Could you check a few things on this model? Use its own coordinates, in mm. A direction names the side the tool comes from. Coordinates: 2 decimals unless noted, no trailing zeros. Loops run counter-clockwise (first coordinate to the right, second up) from the corner with the lowest first, then second, coordinate; pieces in that order, holes last. Notation, with made-up numbers: (-39, 16.5) -> (-28, 16.5) arc R10 cw to (-28, 28.5) -> close; hole circle Ø2 at (-26, 22.5). An arc over 180 degrees is marked (long way). One line per question, with ' | ' between items.
```python
from build123d import *

# Parameters (mm, degrees)
BOSS_EXTRU_1_DEPTH      = 8
CONG_1_R                = 4
ESQUISSE2_R             = 1.25
ENL_V_MAT_EXTRU_1_DEPTH = 8


with BuildPart() as part:
    # Esquisse1 → Boss.-Extru.1 (new body)
    with BuildSketch(Plane.XY):
        with BuildLine():
            Line((9.8, 25), (4.3, 25))
            Line((4.3, 25), (0, 5))
            Line((0, 5), (0, 0))
            Line((0, 0), (50, 0))
            Line((50, 0), (50, 5))
            Line((50, 5), (45.7, 25))
            Line((45.7, 25), (40.2, 25))
            ThreePointArc((40.2, 25), (25, 9.8), (9.8, 25))
        make_face()
    extrude(amount=BOSS_EXTRU_1_DEPTH)

    # Congé1
    cong_1_edges = [part.edges().sort_by_distance(p)[0] for p in [
        (40.2, 25, 4),
        (9.8, 25, 4),
    ]]
    fillet(cong_1_edges, radius=CONG_1_R)

    # Esquisse2 → Enlèv. mat.-Extru.1 (cut)
    with BuildSketch(Plane.XZ):
        with Locations(Location((5, 4, 0), (0, 0, 270))):
            Circle(ESQUISSE2_R)
        with Locations(Location((45, 4, 0), (0, 0, 90))):
            Circle(ESQUISSE2_R)
    extrude(amount=-ENL_V_MAT_EXTRU_1_DEPTH, mode=Mode.SUBTRACT)


solid = part.part
```
Q1. Imagine slicing it at C-C on x = 45. Write out the boundary of the cut face in (y, z).
Values follow:
outline: (0, 0) -> (25, 0) -> (25, 8) -> (0, 8) -> (0, 5.25) -> (8, 5.25) -> (8, 2.75) -> (0, 2.75) -> close
Q2. For pin 1 (0.8 mm diameter, centred on x = 44.5, z = 4.5, fed in from -Y); pin 2 (1 mm diameter, centred on y = 12.5, z = 1.5, fed in from -X) (3 decimals); pin 3 (2 mm diameter, centred on y = 15, z = 4, fed in from +X) (3 decimals), each with a flat end and sliding along its axis, tell me the tip position at first contact or that it passes through.
Values follow:
pin 1: stops at y = 8 | pin 2: stops at x = 1.505 | pin 3: stops at x = 48.065
Q3. Imagine slicing it at D-D on y = 7.5. Write out the boundary of the cut face in (x, z), plus the area to 3 significant figures.
Values follow:
outline: (0.54, 0) -> (49.46, 0) -> (49.46, 8) -> (0.54, 8) -> close; hole circle Ø2.5 at (5, 4); hole circle Ø2.5 at (45, 4) | area: 382 mm2
Q4. For faces 1 (the face through (41.29, 24.13, 4.06)), 2 (the face through (5, 8, 4)), 3 (the face through (45, 25, 4)), which set-ups out of +Z, -Z, +X, -X, +Y, -Y let a thin tool reach every point of the face, with its end or its side?
Values follow:
face 1: +Z, -Z, +Y | face 2: -Y | face 3: +Z, -Z, +X, -X, +Y
Q5. We'd pull the mould along X, two halves only. Please class faces 4 (the face through (50, 2, 4)), 5 (the face through (25, 7, 8)), 6 (the face through (0, 3, 4)), 7 (the face through (3.78, 3.94, 4.27)): released by +X, released by -X, zero draft, split by the parting line, or undercut.
Values follow:
face 4: released by +X | face 5: zero draft | face 6: released by -X | face 7: undercut
Q6. Imagine slicing it at B-B on z = 6. Write out the boundary of the cut face in (x, y), plus the area to 3 significant figures.
Values follow:
outline: (0, 0) -> (50, 0) -> (50, 5) -> (45.7, 25) -> (43.78, 25) arc R4 ccw to (39.87, 21.83) arc R15.2 cw to (10.13, 21.83) arc R4 ccw to (6.22, 25) -> (4.3, 25) -> (0, 5) -> close | area: 796 mm2
Q7. Please list where these lines run through material, in increasing order: L1, parallel to X at y = 2.75, z = 4; L2, parallel to X at y = 6.25, z = 4; L3, parallel to X at y = 12.25, z = 3.5. Write a range as [from, to].
Values follow:
L1: x = [0, 3.75], [6.25, 43.75], [46.25, 50] | L2: x = [0.27, 3.75], [6.25, 43.75], [46.25, 49.73] | L3: x = [1.56, 16.72], [33.28, 48.44]
Q8. Imagine slicing it at A-A on y = 14. Write out the boundary of the cut face in (x, z) (3 decimals).
Values follow:
outline: (1.935, 0) -> (14.51, 0) -> (14.51, 8) -> (1.935, 8) -> close; (35.49, 0) -> (48.065, 0) -> (48.065, 8) -> (35.49, 8) -> close
